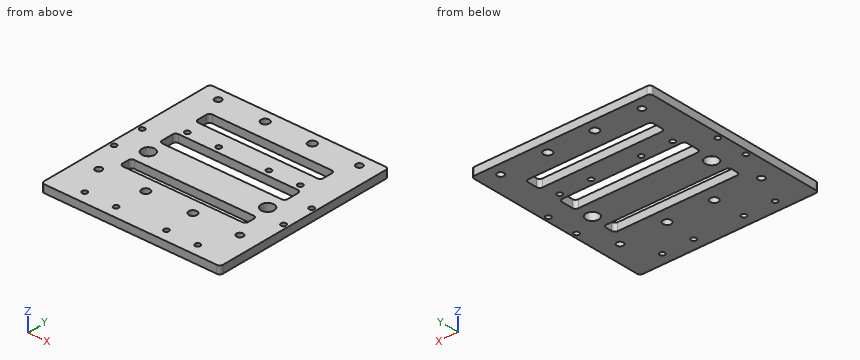
```python
from build123d import *

# Parameters (mm, degrees)
SKETCH_1_W          = 114
SKETCH_1_H          = 120
SKETCH_1_R          = 2.65
SKETCH_1_R_2        = 2.15
EXTRUDE_1_DEPTH     = 5
SKETCH_2_R          = 1.65
CUT_EXTRUDE_1_DEPTH = 83.909589313
SKETCH_3_R          = 4.15
CUT_EXTRUDE_2_DEPTH = 83.909589313
SKETCH_6_R          = 1.65
CUT_EXTRUDE_4_DEPTH = 83.909589313
SKETCH_7_W          = 80
SKETCH_7_H          = 11.5
SKETCH_7_H_2        = 10
SKETCH_7_H_3        = 8
CUT_EXTRUDE_5_DEPTH = 83.909589313
FILLET_1_R          = 2


with BuildPart() as part:
    # 草图1 → 凸台-拉伸1 (new body)
    with BuildSketch(Plane.XY):
        Rectangle(SKETCH_1_W, SKETCH_1_H)
        with Locations((-15, -32.5)):
            Circle(SKETCH_1_R, mode=Mode.SUBTRACT)
        with Locations((15, -32.5)):
            Circle(SKETCH_1_R, mode=Mode.SUBTRACT)
        with Locations((-45, -32.5)):
            Circle(SKETCH_1_R_2, mode=Mode.SUBTRACT)
        with Locations(Location((45, -32.5, 0), (0, 0, 180))):
            Circle(SKETCH_1_R_2, mode=Mode.SUBTRACT)
        with Locations((-45, 52.5)):
            Circle(SKETCH_1_R_2, mode=Mode.SUBTRACT)
        with Locations((-15, 52.5)):
            Circle(SKETCH_1_R, mode=Mode.SUBTRACT)
        with Locations((15, 52.5)):
            Circle(SKETCH_1_R, mode=Mode.SUBTRACT)
        with Locations(Location((45, 52.5, 0), (0, 0, 180))):
            Circle(SKETCH_1_R_2, mode=Mode.SUBTRACT)
    extrude(amount=EXTRUDE_1_DEPTH)

    # 草图2 → 切除-拉伸1 (cut, through all)
    with BuildSketch(Plane.XY.offset(5)):
        with Locations((-16, -52.5)):
            Circle(SKETCH_2_R)
        with Locations((-36, -52.5)):
            Circle(SKETCH_2_R)
        with Locations(Location((16, -52.5, 0), (0, 0, 180))):
            Circle(SKETCH_2_R)
        with Locations(Location((36, -52.5, 0), (0, 0, 180))):
            Circle(SKETCH_2_R)
        with Locations((-16, 20.5)):
            Circle(SKETCH_2_R)
        with Locations((-36, 20.5)):
            Circle(SKETCH_2_R)
        with Locations(Location((16, 20.5, 0), (0, 0, 180))):
            Circle(SKETCH_2_R)
        with Locations(Location((36, 20.5, 0), (0, 0, 180))):
            Circle(SKETCH_2_R)
    extrude(amount=-CUT_EXTRUDE_1_DEPTH, mode=Mode.SUBTRACT)

    # 草图3 → 切除-拉伸2 (cut, through all)
    with BuildSketch(Plane.XY.offset(5)):
        with Locations((-38, -5)):
            Circle(SKETCH_3_R)
        with Locations(Location((38, -5, 0), (0, 0, 180))):
            Circle(SKETCH_3_R)
    extrude(amount=-CUT_EXTRUDE_2_DEPTH, mode=Mode.SUBTRACT)

    # 草图6 → 切除-拉伸4 (cut, through all)
    with BuildSketch(Plane.XY.offset(5)):
        with Locations((54, -11.5)):
            Circle(SKETCH_6_R)
        with Locations((54, 8.5)):
            Circle(SKETCH_6_R)
        with Locations(Location((-54, -11.5, 0), (0, 0, 180))):
            Circle(SKETCH_6_R)
        with Locations(Location((-54, 8.5, 0), (0, 0, 180))):
            Circle(SKETCH_6_R)
    extrude(amount=-CUT_EXTRUDE_4_DEPTH, mode=Mode.SUBTRACT)

    # 草图7 → 切除-拉伸5 (cut, through all)
    with BuildSketch(Plane.XY.offset(5)):
        with Locations((0, 10.75)):
            Rectangle(SKETCH_7_W, SKETCH_7_H)
        with Locations((0, 35.5)):
            Rectangle(SKETCH_7_W, SKETCH_7_H_2)
        with Locations((0, -19)):
            Rectangle(SKETCH_7_W, SKETCH_7_H_3)
    extrude(amount=-CUT_EXTRUDE_5_DEPTH, mode=Mode.SUBTRACT)

    # 圆角1
    fillet_1_edges = [part.edges().sort_by_distance(p)[0] for p in [
        (-40, -23, 2.5),
        (-40, -15, 2.5),
        (40, -15, 2.5),
        (40, -23, 2.5),
        (-40, 30.5, 2.5),
        (-40, 40.5, 2.5),
        (40, 40.5, 2.5),
        (40, 30.5, 2.5),
        (-40, 5, 2.5),
        (-40, 16.5, 2.5),
        (40, 16.5, 2.5),
        (40, 5, 2.5),
        (57, -60, 2.5),
        (-57, -60, 2.5),
        (-57, 60, 2.5),
        (57, 60, 2.5),
    ]]
    fillet(fillet_1_edges, radius=FILLET_1_R)


solid = part.part
```
Can you work these out from the model? Positions are in its coordinate system, mm. Give positions to 0.01 mm unless a question says otherwise; leave off trailing zeros. Order: outer loops, then holes, each group sorted by start corner. A loop starts at its lowest first (then second) coordinate and runs counter-clockwise, first axis right, second up. Notation, with made-up numbers: M 23,46 L 44,46 A20 cw 44,84 Z; hole C 45,42 d5. An arc over 180 degrees is marked long. Write item = value, one per line. Start each with the question number.
Q1. Suppose I cut it at A-A (x = -45). Write out the boundary of the cut face in (y, z), plus the area to 3 significant figures.
Q2. Suppose I cut it at B-B (y = -5). Write out the boundary of the cut face in (x, z), plus the area to 3 significant figures.
Q3. I need wall thicknesses on probe 1 along Y at (x, z) = (-45, 3.35); probe 2 along Y at (x, z) = (-38, 3.4); probe 3 along Y at (x, z) = (-23.5, 2.45). Which ranges of each line are inside material? Lowest first, please. Write a range as [from, to].
Q4. Suppose I cut it at D-D (x = -32). Write out the boundary of the cut face in (y, z).
Q5. Suppose I cut it at C-C (y = 52.5). Write out the boundary of the cut face in (x, z), plus the area to 3 significant figures.
Check result:
q1.outline = M -60,0 L -34.65,0 L -34.65,5 L -60,5 Z; M -30.35,0 L 50.35,0 L 50.35,5 L -30.35,5 Z; M 54.65,0 L 60,0 L 60,5 L 54.65,5 Z
q1.area = 557 mm2
q2.outline = M -57,0 L -42.15,0 L -42.15,5 L -57,5 Z; M -33.85,0 L 33.85,0 L 33.85,5 L -33.85,5 Z; M 42.15,0 L 57,0 L 57,5 L 42.15,5 Z
q2.area = 487 mm2
q3.probe_1 = [-60, -34.65], [-30.35, 50.35], [54.65, 60]
q3.probe_2 = [-60, -23], [-15, -9.15], [-0.85, 5], [16.5, 30.5], [40.5, 60]
q3.probe_3 = [-60, -23], [-15, 5], [16.5, 30.5], [40.5, 60]
q4.outline = M -60,0 L -23,0 L -23,5 L -60,5 Z; M -15,0 L 5,0 L 5,5 L -15,5 Z; M 16.5,0 L 30.5,0 L 30.5,5 L 16.5,5 Z; M 40.5,0 L 60,0 L 60,5 L 40.5,5 Z
q5.outline = M -57,0 L -47.15,0 L -47.15,5 L -57,5 Z; M -42.85,0 L -17.65,0 L -17.65,5 L -42.85,5 Z; M -12.35,0 L 12.35,0 L 12.35,5 L -12.35,5 Z; M 17.65,0 L 42.85,0 L 42.85,5 L 17.65,5 Z; M 47.15,0 L 57,0 L 57,5 L 47.15,5 Z
q5.area = 474 mm2
